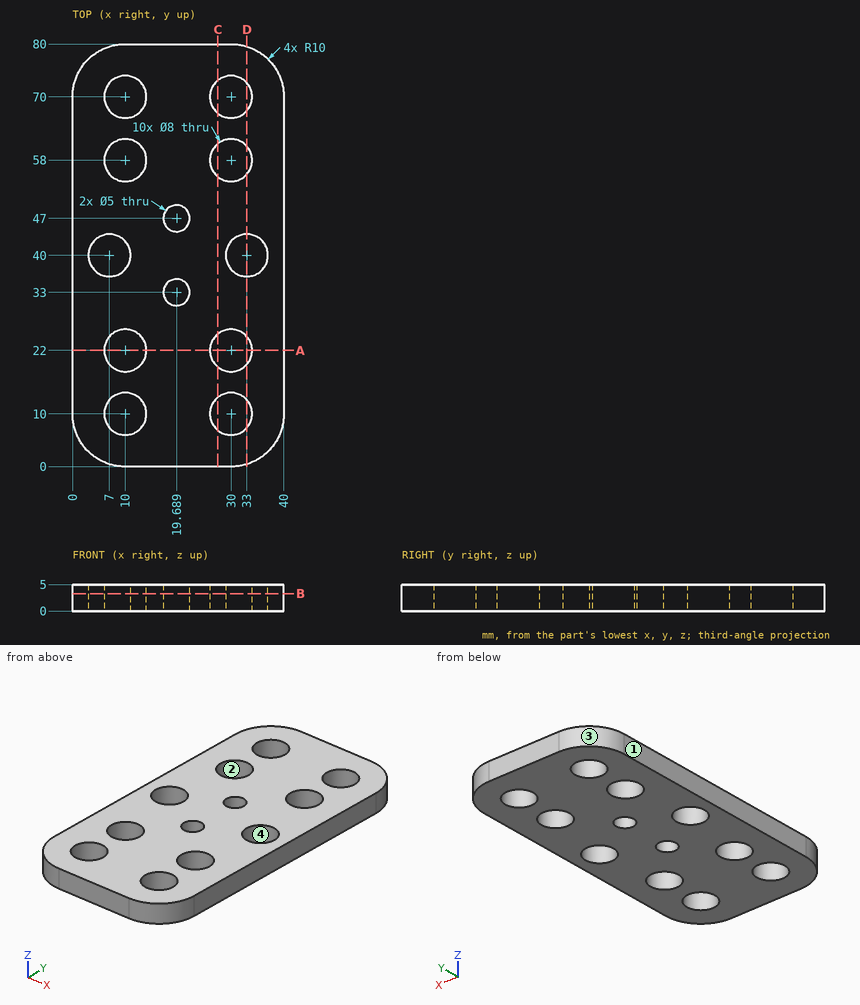
The figure shows three views and two pictorial views of one solid part (mm, origin at its lowest corner). Answer the questions. Give positions to 0.01 mm unless a question says otherwise; leave off trailing zeros. Order: outer loops, then holes, each group sorted by start corner. A loop starts at its lowest first (then second) coordinate and runs counter-clockwise, first axis right, second up. Notation, with made-up numbers: M -39,67 L -3,67 A30 ccw -3,90 Z; hole C 32.25,75.25 d3. An arc over 180 degrees is marked long. Return JSON: item names as keys, results as strings.
Q1. Find section D-D, the plane x = 33. Write down the section's boundary in (y, z) (1 decimal).
Answer below:
{"outline": "M 0.5,0 L 7.4,0 L 7.4,5 L 0.5,5 Z; M 12.6,0 L 19.4,0 L 19.4,5 L 12.6,5 Z; M 24.6,0 L 36,0 L 36,5 L 24.6,5 Z; M 44,0 L 55.4,0 L 55.4,5 L 44,5 Z; M 60.6,0 L 67.4,0 L 67.4,5 L 60.6,5 Z; M 72.6,0 L 79.5,0 L 79.5,5 L 72.6,5 Z"}
Q2. Find the intervals of material crossed by line 1 along X through (y, z) = (56, 2.95) (1 decimal); line 2 along X through (y, z) = (13.5, 1.15) (1 decimal); line 3 along Y through (x, z) = (6.5, 4.1) (1 decimal), in increasing order. Write a range as [from, to].
Answer below:
{"line 1": "x = [0, 6.5], [13.5, 26.5], [33.5, 40]", "line 2": "x = [0, 8.1], [11.9, 28.1], [31.9, 40]", "line 3": "y = [0.6, 8.1], [11.9, 20.1], [23.9, 36], [44, 56.1], [59.9, 68.1], [71.9, 79.4]"}
Q3. This flat-tipped pin is pushed along its axis until it touches: pin 1 (5 mm diameter, centred on x = 30, y = 70, fed in from +Z). Where does it stop, or does it pass through?
Answer below:
{"pin 1": "passes through"}
Q4. The mould has two halves that part along Y. Classify the marked faces 1, 2, 3 and 4: pulls with the +Y half, pulls with the -Y half, needs draft (parallel to the pull), parting line crosses it, or undercut.
Answer below:
{"face 1": "needs draft", "face 2": "undercut", "face 3": "pulls with the +Y half", "face 4": "undercut"}
Q5. Find section B-B, the plane z = 3.3. State how many separate pieces and enclosed holes the cut face has, and give its area (3 significant figures).
Answer below:
{"separate pieces": "1", "enclosed holes": "12", "area": "2,570 mm^2"}
Q6. Find section A-A, the plane y = 22. Write down the section's boundary in (x, z).
Answer below:
{"outline": "M 0,0 L 6,0 L 6,5 L 0,5 Z; M 14,0 L 26,0 L 26,5 L 14,5 Z; M 34,0 L 40,0 L 40,5 L 34,5 Z"}
Q7. Find section C-C, the plane x = 27.5. Write down the section's boundary in (y, z), and give its area (3 significant figures).
Answer below:
{"outline": "M 0,0 L 6.88,0 L 6.88,5 L 0,5 Z; M 13.12,0 L 18.88,0 L 18.88,5 L 13.12,5 Z; M 25.12,0 L 54.88,0 L 54.88,5 L 25.12,5 Z; M 61.12,0 L 66.88,0 L 66.88,5 L 61.12,5 Z; M 73.12,0 L 80,0 L 80,5 L 73.12,5 Z", "area": "275 mm^2"}
